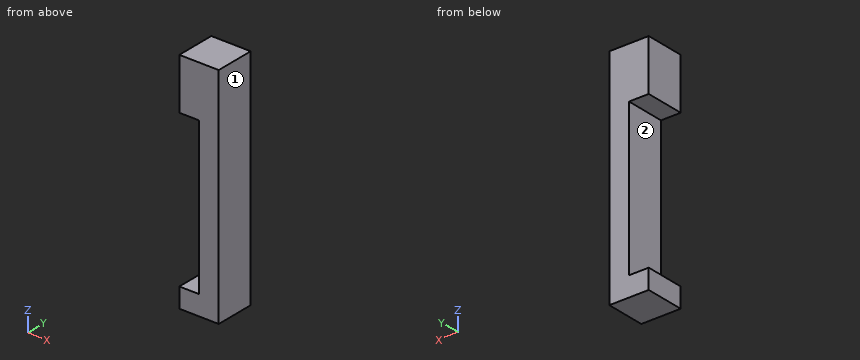
```python
from build123d import *

# Parameters (mm, degrees)
SKETCH1_W           = 25.4
SKETCH1_H           = 33.02
SKETCH1_W_2         = 12.7
SKETCH1_H_2         = 12.7
BOSS_EXTRUDE1_DEPTH = 25.4


with BuildPart() as part:
    # Sketch1 → Boss-Extrude1 (new body)
    with BuildSketch(Plane(origin=(0, 0, 0), x_dir=(1, 0, 0), z_dir=(0, 1, 0))):
        with Locations((-12.7, 16.51)):
            Rectangle(SKETCH1_W, SKETCH1_H)
        Polygon((-12.7, 33.02), (0, 33.02), (0, 144.78), (-12.7, 144.78), (-12.7, 132.08), align=None)
        with Locations((-19.05, 138.43)):
            Rectangle(SKETCH1_W_2, SKETCH1_H_2)
    extrude(amount=BOSS_EXTRUDE1_DEPTH)


solid = part.part
```
Design review of the part built by this model. Coordinates are the model's own, in mm. Face numbers are marked on the shaded views. A direction names the side the tool comes from. Coordinates: 2 decimals unless noted, no trailing zeros. Order: outer loops, then holes, each group sorted by start corner. A loop starts at its lowest first (then second) coordinate and runs counter-clockwise, first axis right, second up. Notation, with made-up numbers: (-15.5, 54) -> (28.5, 54) arc R37 cw to (28.5, 93) -> close; hole circle Ø6 at (42, 67). An arc over 180 degrees is marked (long way). One line per item, written item: value. Start each with the question number.
Q1. Take a section at C-C, the plane z = -59. State the section outline as (x, y) points, then the cut area to 3 significant figures.
Q2. Take a section at B-B, the plane y = 23.75. State the section outline as (x, z) points, then the cut area to 3 significant figures.
Q3. For probe 1 along Z at (x, y) = (-16.75, 21); probe 2 along X at (y, z) = (20.25, -82.5), list the stretches that pass through material, from the lowest coordinate up.
Q4. Take a section at A-A, the plane x = -14.5. State the section outline as (y, z) points, then the cut area to 3 significant figures.
Q5. Tool access review of the marked faces 1 and 2: name each direction out of +Z, -Z, +X, -X, +Y, -Y from which nothing blocks a thin tool from reaching the whole face with its end or side.
Values follow:
1. outline: (-12.7, 0) -> (0, 0) -> (0, 25.4) -> (-12.7, 25.4) -> close
1. area: 323 mm2
2. outline: (-25.4, -144.78) -> (0, -144.78) -> (0, 0) -> (-25.4, 0) -> (-25.4, -33.02) -> (-12.7, -33.02) -> (-12.7, -132.08) -> (-25.4, -132.08) -> close
2. area: 2,420 mm2
3. probe 1: z = -144.78 to -132.08, -33.02 to 0
3. probe 2: x = -12.7 to 0
4. outline: (0, -144.78) -> (25.4, -144.78) -> (25.4, -132.08) -> (0, -132.08) -> close; (0, -33.02) -> (25.4, -33.02) -> (25.4, 0) -> (0, 0) -> close
4. area: 1,160 mm2
5. face 1: +Z, -Z, +X, +Y, -Y
5. face 2: -X, +Y, -Y
